Check sheet for the modelled part. Datum: model origin and axes. Units: mm. A direction names the side the tool comes from. Give positions to 0.01 mm unless a question says otherwise; leave off trailing zeros. Write each loop counter-clockwise with the first axis right and the second up, starting at its lowest first coordinate (ties: lowest second). Pieces come first, ordered by that corner, then holes. Notation, with made-up numbers: M 47,37.25 L 95,37.25 A36 cw 95,71.25 Z; hole C 68,51.5 d7. An arc over 180 degrees is marked long. Write item = value, one per line. Start each with the question number.
1) Gauge pin test, flat ends, axial feed: pin 1 (2 mm diameter, centred on x = -61.5, z = -11, fed in from +Y); pin 2 (1 mm diameter, centred on y = 15.5, z = 70, fed in from -X); pin 3 (10 mm diameter, centred on x = 53, z = -56.5, fed in from +Y); pin 4 (5 mm diameter, centred on y = 11, z = 44, fed in from +X). Record the tip position at first contact, or that the pin passes through.
2) Draft check along X on faces 1 (the face through (60, 7, 1)), 2 (the face through (-46, -5, 6)), 3 (the face through (-89.25, 6, -75)). Enter one of: pulls with the +X half, pulls with the -X half, needs draft (parallel to the pull), parting line crosses it, or undercut.
3) Scan lines: L1, parallel to X at y = 2.75, z = -63; L2, parallel to Z at x = -70, y = -1.75; L3, parallel to X at y = 8.75, z = 1.5. Record each from-to range of solid material in increasing order.
4) Sectioned sample at C-C, the plane y = 2.25. Count the separate pieces of the cut face and the enclosed holes in it, then the cut area to 3 significant figures.
5) Sectioned sample at B-B, the plane x = 72.5. Record the cut outline in (y, z), then the cut area to 3 significant figures.
6) Set-up check for faces 4 (the face through (-95, 12.5, 75)), 5 (the face through (0.63, -1.99, 65.35)), 6 (the face through (-35, 7, 1)), 7 (the face through (-86.5, 9, -75)): record each of +Z, -Z, +X, -X, +Y, -Y from which the full face is reachable in a straight line by a thin tool's end or side.
7) Sectioned sample at D-D, the plane x = 4. Record the cut outline in (y, z), then the cut area to 3 significant figures.
8) Sectioned sample at A-A, the plane z = 14. Record the cut outline in (x, y).
from build123d import *

# Parameters (mm, degrees)
BOSS_EXTRUDE1_DEPTH      = 19.25
BOSS_EXTRUDE1_DEPTH_BACK = 5
SKETCH1_W                = 70
SKETCH1_H                = 125
SKETCH2_W                = 15
SKETCH2_H                = 25
BOSS_EXTRUDE2_DEPTH      = 5
SKETCH3_W                = 12.25
SKETCH3_H                = 25
BOSS_EXTRUDE3_DEPTH      = 12.5
FILLET1_R                = 10


with BuildPart() as part:
    # Sketch1 → Boss-Extrude1 (new, two sides: drawn at the far end of the back side and taken through both)
    with BuildSketch(Plane(origin=(0, 0, 0), x_dir=(1, 0, 0), z_dir=(0, 1, 0)).offset(-BOSS_EXTRUDE1_DEPTH_BACK)):
        Polygon((-60, 62.5), (-60, -62.5), (-86.5, -62.5), (-86.5, -87.5), (86.5, -87.5), (86.5, -62.5), (60, -62.5), (60, 62.5), (86.5, 62.5), (86.5, 87.5), (-86.5, 87.5), (-86.5, 62.5), align=None)
        Rectangle(SKETCH1_W, SKETCH1_H, mode=Mode.SUBTRACT)
    extrude(amount=BOSS_EXTRUDE1_DEPTH + BOSS_EXTRUDE1_DEPTH_BACK)

    # Sketch2 → Boss-Extrude2 (add)
    with BuildSketch(Plane(origin=(0, -5, 0), x_dir=(1, 0, 0), z_dir=(0, 1, 0))):
        with Locations((-94, 75)):
            Rectangle(SKETCH2_W, SKETCH2_H)
        with Locations((94, 75)):
            Rectangle(SKETCH2_W, SKETCH2_H)
        with Locations((-94, -75)):
            Rectangle(SKETCH2_W, SKETCH2_H)
        with Locations((94, -75)):
            Rectangle(SKETCH2_W, SKETCH2_H)
    extrude(amount=BOSS_EXTRUDE2_DEPTH)

    # Sketch3 → Boss-Extrude3 (add)
    with BuildSketch(Plane(origin=(0, 0, 0), x_dir=(1, 0, 0), z_dir=(0, 1, 0))):
        with Locations((-95.375, 75)):
            Rectangle(SKETCH3_W, SKETCH3_H)
        with Locations((95.375, 75)):
            Rectangle(SKETCH3_W, SKETCH3_H)
        with Locations((-95.375, -75)):
            Rectangle(SKETCH3_W, SKETCH3_H)
        with Locations((95.375, -75)):
            Rectangle(SKETCH3_W, SKETCH3_H)
    extrude(amount=BOSS_EXTRUDE3_DEPTH)

    # Fillet1
    fillet1_edges = [part.edges().sort_by_distance(p)[0] for p in [
        (0, 19.25, 62.5),
        (60, 19.25, 0),
        (35, 19.25, 0),
        (-60, 19.25, 0),
        (-35, 19.25, 0),
        (0, 19.25, -62.5),
        (0, -5, 62.5),
        (-35, -5, 0),
        (0, -5, -62.5),
        (35, -5, 0),
        (60, -5, 0),
        (-60, -5, 0),
    ]]
    fillet(fillet1_edges, radius=FILLET1_R)


solid = part.part
Data:
q1.pin_1 = through
q1.pin_2 = -86.5
q1.pin_3 = 19.25
q1.pin_4 = 60
q2.face_1 = pulls with the +X half
q2.face_2 = needs draft
q2.face_3 = undercut
q3.L1 = -101.5 to -89.25, -86.5 to 86.5, 89.25 to 101.5
q3.L2 = -87.5 to -62.5, 62.5 to 87.5
q3.L3 = -60 to -35, 35 to 60
q4.separate_pieces = 5
q4.enclosed_holes = 1
q4.area = 15,900 mm2
q5.outline = M -5,-87.5 L 19.25,-87.5 L 19.25,-62.5 L -5,-62.5 Z; M -5,62.5 L 19.25,62.5 L 19.25,87.5 L -5,87.5 Z
q5.area = 1,210 mm2
q6.face_4 = +Z, -Z, -X, +Y
q6.face_5 = -Y
q6.face_6 = +Y, -Y
q6.face_7 = +Z, -Z, +Y
q7.outline = M -5,-87.5 L 19.25,-87.5 L 19.25,-72.5 A10 ccw 9.25,-62.5 L 5,-62.5 A10 ccw -5,-72.5 Z; M -5,72.5 A10 ccw 5,62.5 L 9.25,62.5 A10 ccw 19.25,72.5 L 19.25,87.5 L -5,87.5 Z
q7.area = 1,130 mm2
q8.outline = M -60,5 A10 ccw -50,-5 L -45,-5 A10 ccw -35,5 L -35,9.25 A10 ccw -45,19.25 L -50,19.25 A10 ccw -60,9.25 Z; M 35,5 A10 ccw 45,-5 L 50,-5 A10 ccw 60,5 L 60,9.25 A10 ccw 50,19.25 L 45,19.25 A10 ccw 35,9.25 Z
